Read the model definition and answer for the solid it produces. Units are mm, in the model's axes. Face numbers are marked on the shaded views. A direction names the side the tool comes from. Give positions to 0.01 mm unless a question says otherwise; leave off trailing zeros. Loops run counter-clockwise (first coordinate to the right, second up) from the corner with the lowest first, then second, coordinate; pieces in that order, holes last. Notation, with made-up numbers: (-0.75, 47.5) -> (45.25, 47.5) arc R10 ccw to (45.25, 51.5) -> close; hole circle Ø10 at (11, 77.5). An arc over 180 degrees is marked (long way). Return JSON: item names as keys, results as strings. Group by question number.
from build123d import *

# Parameters (mm, degrees)
SKETCH1_W           = 88
SKETCH1_H           = 41
BOSS_EXTRUDE1_DEPTH = 3
BOSS_EXTRUDE2_DEPTH = 3
BOSS_EXTRUDE3_DEPTH = 60
BOSS_EXTRUDE4_DEPTH = 1
FILLET1_R           = 10
SKETCH5_W           = 32
SKETCH5_H           = 3
BOSS_EXTRUDE5_DEPTH = 8
FILLET2_R           = 10
FILLET6_R           = 1
FILLET12_R          = 3
SKETCH6_W           = 81.912475118
SKETCH6_H           = 4
BOSS_EXTRUDE6_DEPTH = 8
SKETCH7_R           = 1.5
CUT_EXTRUDE1_DEPTH  = 3


with BuildPart() as part:
    # Sketch1 → Boss-Extrude1 (new body)
    with BuildSketch(Plane.XY):
        with Locations((44, 20.5)):
            Rectangle(SKETCH1_W, SKETCH1_H)
    extrude(amount=BOSS_EXTRUDE1_DEPTH)

    # Sketch2 → Boss-Extrude2 (add)
    with BuildSketch(Plane.XY.offset(3)):
        Polygon((0, 0), (88, 0), (82, -35), (6, -35), align=None)
    extrude(amount=-BOSS_EXTRUDE2_DEPTH)

    # Sketch3 → Boss-Extrude3 (add)
    with BuildSketch(Plane(origin=(0, 0, 0), x_dir=(-1, 0, 0), z_dir=(0, 0, -1))):
        Polygon((-82, -35), (-88, 0), (-84.956237559, 0), (-79.470523274, -32), (-60, -32), (-60, -35), align=None)
        Polygon((-28, -35), (-6, -35), (0, 0), (-3.043762441, 0), (-8.529476726, -32), (-28, -32), align=None)
    extrude(amount=BOSS_EXTRUDE3_DEPTH)

    # Sketch4 → Boss-Extrude4 (add)
    with BuildSketch(Plane(origin=(0, 41, 0), x_dir=(1, 0, 0), z_dir=(0, 1, 0))):
        Polygon((0, -3), (-7, 21), (-7, 54), (27, 54), (27, 9), (61, 9), (61, 54), (95, 54), (95, 21), (88, -3), align=None)
    extrude(amount=BOSS_EXTRUDE4_DEPTH)

    # Fillet1
    fillet1_edges = [part.edges().sort_by_distance(p)[0] for p in [
        (61, 41.5, -9),
        (27, 41.5, -9),
    ]]
    fillet(fillet1_edges, radius=FILLET1_R)

    # Sketch5 → Boss-Extrude5 (add)
    with BuildSketch(Plane(origin=(0, 0, 0), x_dir=(-1, 0, 0), z_dir=(0, 0, -1))):
        with Locations((-44, -33.5)):
            Rectangle(SKETCH5_W, SKETCH5_H)
    extrude(amount=BOSS_EXTRUDE5_DEPTH)

    # Fillet2
    fillet2_edges = [part.edges().sort_by_distance(p)[0] for p in [
        (60, -33.5, -8),
        (28, -33.5, -8),
    ]]
    fillet(fillet2_edges, radius=FILLET2_R)

    # Fillet6
    fillet6_edges = [part.edges().sort_by_distance(p)[0] for p in [
        (44, 42, 3),
    ]]
    fillet(fillet6_edges, radius=FILLET6_R)

    # Fillet12
    fillet12_edges = [part.edges().sort_by_distance(p)[0] for p in [
        (85, -17.5, -60),
        (60, -33.5, -60),
        (28, -33.5, -60),
        (3, -17.5, -60),
        (3, -17.5, 3),
        (85, -17.5, 3),
        (71, -35, -60),
        (17, -35, -60),
        (82, -35, -28.5),
        (6, -35, -28.5),
        (44, -35, 3),
    ]]
    fillet(fillet12_edges, radius=FILLET12_R - 0.0001)  # a hair under: the kernel refuses the full size

    # Sketch6 → Boss-Extrude6 (add)
    with BuildSketch(Plane(origin=(0, 0, 0), x_dir=(-1, 0, 0), z_dir=(0, 0, -1))):
        with Locations((-44, -2)):
            Rectangle(SKETCH6_W, SKETCH6_H)
    extrude(amount=BOSS_EXTRUDE6_DEPTH)

    # Sketch7 → Cut-Extrude1 (cut)
    with BuildSketch(Plane(origin=(0, 0, 0), x_dir=(-1, 0, 0), z_dir=(0, 0, -1))):
        with Locations((-12, 32.5)):
            Circle(SKETCH7_R)
        with Locations(Location((-76, 32.5, 0), (0, 0, 180))):
            Circle(SKETCH7_R)
        with Locations((-76, 8.5)):
            Circle(SKETCH7_R)
        with Locations(Location((-12, 8.5, 0), (0, 0, 180))):
            Circle(SKETCH7_R)
    extrude(amount=-CUT_EXTRUDE1_DEPTH, mode=Mode.SUBTRACT)


solid = part.part
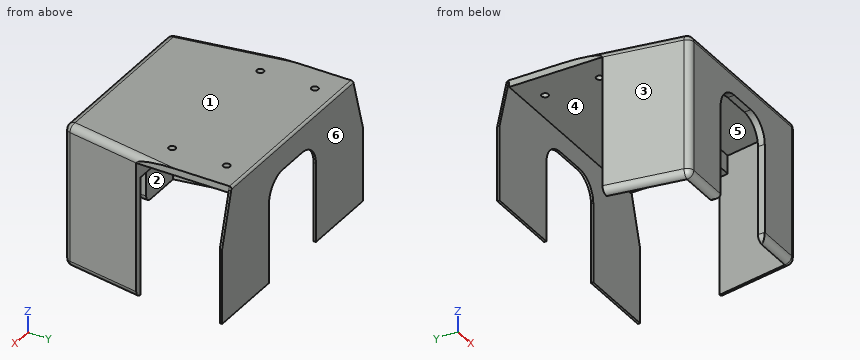
1. Section B-B on z = -44.5 is taken. Determine the outline of the cut face in (x, y), then the cut area to 3 significant figures.
2. Section C-C on x = 12 is taken. State how many separate pieces and enclosed holes the cut face has, then the cut area to 3 significant figures.
3. Section A-A on y = 32.5 is taken. Determine the outline of the cut face in (x, z).
4. Which of the six approach directions +Z, -Z, +X, -X, +Y, -Y give full straight-line access (tool end or side, diameter ignored) to the marked faces 4, 5 and 6?
5. Determine the mould class of the marked faces 1, 2 and 3 for opening direction X: pulls with the +X half, pulls with the -X half, needs draft (parallel to the pull), parting line crosses it, or undercut.
6. Flat-ended cylindrical pins translate along their axes: pin 1 Ø1.1 at (x, y) = (43.5, 41.5) entering from -Z; pin 2 Ø1.5 at (y, z) = (12, 1) entering from -X; pin 3 Ø1.5 at (y, z) = (-0.5, -15.5) entering from +X; pin 4 Ø2.5 at (x, y) = (12, 32.5) entering from -Z. Find the tip coordinate at first contact, or state that the pin passes through.
7. Straight lines are drawn through the part: line 1 (Y direction, x = 76, z = 1); line 2 (X direction, y = 32, z = 1); line 3 (Y direction, x = 76, z = 0.85). For each, find the intervals that lie inside material, in ascending order. Write a range as from..to.
8. Section D-D on z = -4 is taken. Determine the outline of the cut face in (x, y).
Completed:
{
 "1": {"outline": "(-7, 41) -> (27, 41) -> (27, 42) -> (-7, 42) -> close; (0, 0) -> (5.57, -32.51) arc R3 ccw to (8.53, -35) -> (28, -35) -> (28, -32) -> (8.53, -32) -> (3.04, 0) -> close; (60, -35) -> (79.47, -35) arc R3 ccw to (82.43, -32.51) -> (88, 0) -> (84.96, 0) -> (79.47, -32) -> (60, -32) -> close; (61, 41) -> (95, 41) -> (95, 42) -> (61, 42) -> close", "area": "394 mm²"},
 "2": {"separate pieces": "3", "enclosed holes": "0", "area": "475 mm²"},
 "3": {"outline": "(0, 0) -> (10.5, 0) -> (10.5, 3) -> (0, 3) -> close; (13.5, 0) -> (74.5, 0) -> (74.5, 3) -> (13.5, 3) -> close; (77.5, 0) -> (88, 0) -> (88, 3) -> (77.5, 3) -> close"},
 "4": {"face 4": "-Z, +X, -X", "face 5": "-Z", "face 6": "+Z, -Z, +X, -X, +Y"},
 "5": {"face 1": "needs draft", "face 2": "undercut", "face 3": "pulls with the -X half"},
 "6": {"pin 1": "stops at z = -9", "pin 2": "stops at x = 0", "pin 3": "stops at x = 88", "pin 4": "passes through"},
 "7": {"line 1": "y = -34.83..7, 10..31, 34..42", "line 2": "x = 0..10.59, 13.41..74.59, 77.41..88", "line 3": "y = -34.88..7, 10..31, 34..42"},
 "8": {"outline": "(-2.04, 41) -> (90.04, 41) -> (90.04, 42) -> (-2.04, 42) -> close; (0, 0) -> (5.57, -32.51) arc R3 ccw to (8.53, -35) -> (79.47, -35) arc R3 ccw to (82.43, -32.51) -> (88, 0) -> close; hole (3.73, -4) -> (8.53, -32) -> (79.47, -32) -> (84.27, -4) -> close"}
}
